Geometry: final body of the model. Coordinates: model frame, mm. Face numbers are marked on the shaded views. A direction names the side the tool comes from. Give positions to 0.01 mm unless a question says otherwise; leave off trailing zeros. Order: outer loops, then holes, each group sorted by start corner. A loop starts at its lowest first (then second) coordinate and runs counter-clockwise, first axis right, second up. Notation, with made-up numbers: M 15,65 L 36,65 A14 ccw 36,74 Z; hole C 70,60.5 d10. An arc over 180 degrees is marked long. Use CSV: the item, a comma, the result in double quotes.
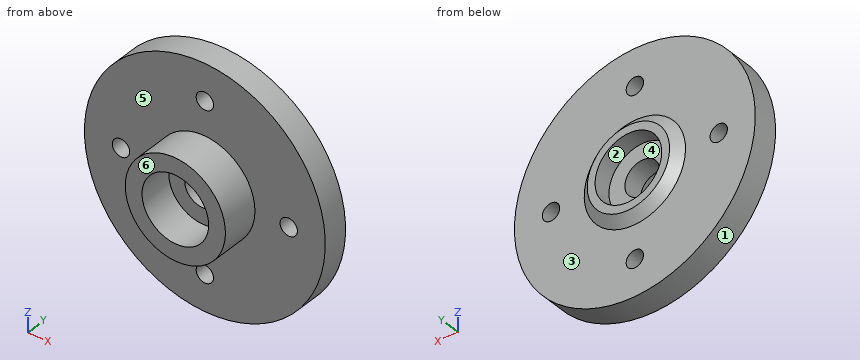
```python
from build123d import *

# Parameters (mm, degrees)
SKETCH_2_R            = 0.75
CUT_EXTRUDE_619_DEPTH = 16.681077769


with BuildPart() as part:
    # 草图1 → 旋转1 (revolve)
    with BuildSketch(Plane.XY, mode=Mode.PRIVATE) as revolve_1_sk:
        Polygon((-2.88, 0), (-2.88, 2.9), (-1.5, 2.9), (-1.5, 4.6), (-2.88, 4.6), (-2.88, 6.1), (-3.56, 6.1), (-4.38, 5.4), (-10.41, 5.4), (-10.41, 3.2), (-4.33, 3.2), (-4.33, 0), align=None)
    revolve(revolve_1_sk.sketch.rotate(Axis((0, 0, 0), (0, 1, 0)), 270), axis=Axis((0, 0, 0), (0, 1, 0)))

    # 草图2 → Cut-Extrude 619 (cut, through all)
    with BuildSketch(Plane(origin=(0, 5.4, 0), x_dir=(1, 0, 0), z_dir=(0, 1, 0))):
        with Locations(Location((0, 7.25, 0), (0, 0, 270))):
            Circle(SKETCH_2_R)
        with Locations(Location((7.25, 0, 0), (0, 0, 270))):
            Circle(SKETCH_2_R)
        with Locations(Location((0, -7.25, 0), (0, 0, 270))):
            Circle(SKETCH_2_R)
        with Locations(Location((-7.25, 0, 0), (0, 0, 270))):
            Circle(SKETCH_2_R)
    extrude(amount=-CUT_EXTRUDE_619_DEPTH, mode=Mode.SUBTRACT)


solid = part.part
```
1. Section A-A, the plane x = 0. Give the number of separate pieces and of enclosed holes in the cut face, plus the area to 3 significant figures.
Answer:
separate pieces,"4"
enclosed holes,"0"
area,"42.0 mm2"
2. Section D-D, the plane y = 5.75. Return the cut outline in (x, z), plus the area to 3 significant figures.
Answer:
outline,"C 0,0 d7.94; hole C 0,0 d5.76"
area,"23.5 mm2"
3. Pin query (flat end, axial travel): pin 1 Ø0.9 at (x, z) = (7.25, 0) entering from -Y; pin 2 Ø1 at (y, z) = (3, -1.5) entering from +X; pin 3 Ø1.5 at (x, y) = (-2.5, 4) entering from -Z; pin 4 Ø1.5 at (y, z) = (5, 1.5) entering from -X. Return the tip coordinate at first contact, or that it passes through.
Answer:
pin 1,"through"
pin 2,"x = 10.36"
pin 3,"z = -10.26"
pin 4,"x = -10.38"
4. Reachability of the marked faces 4, 5 and 6 from +Z, -Z, +X, -X, +Y, -Y: full face, straight path, thin tool, end or side. Return the list, or none.
Answer:
face 4,"+Y"
face 5,"-Y"
face 6,"+Z, -Z, +X, -X, -Y"
5. Section C-C, the plane z = -7.25. Return the cut outline in (x, y).
Answer:
outline,"M -7.47,3.2 L -0.75,3.2 L -0.75,5.4 L -7.47,5.4 Z; M 0.75,3.2 L 7.47,3.2 L 7.47,5.4 L 0.75,5.4 Z"
6. Pull-direction query (X, two-part tool) for the marked faces 1, 2 and 3; classes: +X half, -X half, draft (parallel to the pull), parting line (faces both ways), or undercut.
Answer:
face 1,"parting line"
face 2,"undercut"
face 3,"draft"
7. Line query: line 1 (X direction, y = 3.65, z = 0); line 2 (X direction, y = 4.9, z = 0); line 3 (X direction, y = 1.2, z = 0). Output: solid intervals per line, ascending.
Answer:
line 1,"-10.41 to -8, -6.5 to -1.5, 1.5 to 6.5, 8 to 10.41"
line 2,"-10.41 to -8, -6.5 to -2.88, 2.88 to 6.5, 8 to 10.41"
line 3,"-4.33 to -2.88, 2.88 to 4.33"
